```python
from build123d import *

# Parameters (mm, degrees)
BOX002_W          = 1
BOX002_H          = 6.4
BOX002_DEPTH      = 1.5
BOX006_W          = 10
BOX006_H          = 4.37
BOX006_DEPTH      = 12
BOX005_W          = 10
BOX005_H          = 4.37
BOX005_DEPTH      = 12
CYLINDER008_R     = 0.59
CYLINDER008_DEPTH = 50
CYLINDER009_R     = 0.59
CYLINDER009_DEPTH = 50
CYLINDER007_R     = 0.59
CYLINDER007_DEPTH = 50
BOX003_W          = 10
BOX003_H          = 4.37
BOX003_DEPTH      = 26
BOX004_W          = 10
BOX004_H          = 4.37
BOX004_DEPTH      = 26
BOX001_W          = 10
BOX001_H          = 5.5
BOX001_DEPTH      = 27
CYLINDER006_R     = 1.695
CYLINDER006_DEPTH = 20
CYLINDER003_R     = 1.1
CYLINDER003_DEPTH = 2
BOX_W             = 2
BOX_H             = 10
BOX_DEPTH         = 27.9
CYLINDER004_R     = 3
CYLINDER004_DEPTH = 27.4
CYLINDER005_R     = 1
CYLINDER005_DEPTH = 5.5
CYLINDER002_R     = 0.75
CYLINDER002_DEPTH = 6.2
CYLINDER001_R     = 2.5
CYLINDER001_DEPTH = 18
CYLINDER_R        = 2.2
CYLINDER_DEPTH    = 21.5


with BuildPart() as obj1:
    # Box002 → Box002 (new body)
    with BuildSketch(Plane(origin=(-0.5, -3.2, 21.5), x_dir=(1, 0, 0), z_dir=(0, 0, 1))):
        with Locations((0.5, 3.2)):
            Rectangle(BOX002_W, BOX002_H)
    extrude(amount=BOX002_DEPTH)


with BuildPart() as obj2:
    # Box006 → Box006 (new body)
    with BuildSketch(Plane(origin=(-10.25, -2.19, 36.77), x_dir=(1, 0, 0), z_dir=(0, 0, 1))):
        with Locations((5, 2.185)):
            Rectangle(BOX006_W, BOX006_H)
    extrude(amount=BOX006_DEPTH)


with BuildPart() as fusion004:
    # Box005 → Box005 (new body)
    with BuildSketch(Plane(origin=(0.25, -2.19, 36.77), x_dir=(1, 0, 0), z_dir=(0, 0, 1))):
        with Locations((5, 2.185)):
            Rectangle(BOX005_W, BOX005_H)
    extrude(amount=BOX005_DEPTH)

    # Fusion004: union obj2
    add(obj2.part)


with BuildPart() as fusion004_1:
    # Fusion004 placement: moved
    add(fusion004.part.moved(Location((0, 0, 1))))


with BuildPart() as m1_6_thread2:
    # Cylinder008 → Cylinder008 (new body)
    with BuildSketch(Plane(origin=(-4, 0, 29.41), x_dir=(0, 0, -1), z_dir=(1, 0, 0))):
        Circle(CYLINDER008_R)
    extrude(amount=CYLINDER008_DEPTH)


with BuildPart() as m1_6_thread3:
    # Cylinder009 → Cylinder009 (new body)
    with BuildSketch(Plane(origin=(-4, 0, 27.41), x_dir=(0, 0, -1), z_dir=(1, 0, 0))):
        Circle(CYLINDER009_R)
    extrude(amount=CYLINDER009_DEPTH)


with BuildPart() as mirrormountingholes:
    # Cylinder007 → Cylinder007 (new body)
    with BuildSketch(Plane(origin=(-4, 0, 31.405), x_dir=(0, 0, -1), z_dir=(1, 0, 0))):
        Circle(CYLINDER007_R)
    extrude(amount=CYLINDER007_DEPTH)

    # Fusion003: union M1_6__Thread2, M1_6__Thread3
    add(m1_6_thread2.part)
    add(m1_6_thread3.part)


with BuildPart() as obj3:
    # Box003 → Box003 (new body)
    with BuildSketch(Plane(origin=(0.5, -2.19, 23), x_dir=(1, 0, 0), z_dir=(0, 0, 1))):
        with Locations((5, 2.185)):
            Rectangle(BOX003_W, BOX003_H)
    extrude(amount=BOX003_DEPTH)


with BuildPart() as mirrorgrooves:
    # Box004 → Box004 (new body)
    with BuildSketch(Plane(origin=(-10.5, -2.19, 23), x_dir=(1, 0, 0), z_dir=(0, 0, 1))):
        with Locations((5, 2.185)):
            Rectangle(BOX004_W, BOX004_H)
    extrude(amount=BOX004_DEPTH)

    # Fusion002: union obj3
    add(obj3.part)


with BuildPart() as obj4:
    # Box001 → Box001 (new body)
    with BuildSketch(Plane(origin=(1, -2.57, 21), x_dir=(1, 0, 0), z_dir=(0, 0, 1))):
        with Locations((5, 2.75)):
            Rectangle(BOX001_W, BOX001_H)
    extrude(amount=BOX001_DEPTH)


with BuildPart() as probehole:
    # Cylinder006 → Cylinder006 (new body)
    with BuildSketch(Plane(origin=(-4, 0, 35.2), x_dir=(0, 0, -1), z_dir=(1, 0, 0))):
        Circle(CYLINDER006_R)
    extrude(amount=CYLINDER006_DEPTH)


with BuildPart() as beamhole:
    # Cylinder003 → Cylinder003 (new body)
    with BuildSketch(Plane(origin=(-1, 0, 35.2), x_dir=(0, 0, -1), z_dir=(1, 0, 0))):
        Circle(CYLINDER003_R)
    extrude(amount=CYLINDER003_DEPTH)


with BuildPart() as obj5:
    # Box → Box (new body)
    with BuildSketch(Plane(origin=(-1, -5, 21), x_dir=(1, 0, 0), z_dir=(0, 0, 1))):
        with Locations((1, 5)):
            Rectangle(BOX_W, BOX_H)
    extrude(amount=BOX_DEPTH)


with BuildPart() as cut004:
    # Cylinder004 → Cylinder004 (new body)
    with BuildSketch(Plane.XY.offset(21.5)):
        Circle(CYLINDER004_R)
    extrude(amount=CYLINDER004_DEPTH)

    # Common: intersect obj5
    add(obj5.part, mode=Mode.INTERSECT)

    # Cut001: cut BeamHole
    add(beamhole.part, mode=Mode.SUBTRACT)

    # Cut003: cut ProbeHole
    add(probehole.part, mode=Mode.SUBTRACT)

    # Cut004: cut obj4
    add(obj4.part, mode=Mode.SUBTRACT)


with BuildPart() as zylinder005:
    # Cylinder005 → Cylinder005 (new body)
    with BuildSketch(Plane.XY.offset(-0.5)):
        Circle(CYLINDER005_R)
    extrude(amount=CYLINDER005_DEPTH)


with BuildPart() as zylinder002:
    # Cylinder002 → Cylinder002 (new body)
    with BuildSketch(Plane(origin=(-3.25, 0, 2.95), x_dir=(0, 0, -1), z_dir=(1, 0, 0))):
        Circle(CYLINDER002_R)
    extrude(amount=CYLINDER002_DEPTH)


with BuildPart() as zylinder001:
    # Cylinder001 → Cylinder001 (new body)
    with BuildSketch(Plane.XY.offset(5)):
        Circle(CYLINDER001_R)
    extrude(amount=CYLINDER001_DEPTH)


with BuildPart() as fusion005:
    # Cylinder → Cylinder (new body)
    with BuildSketch(Plane.XY.offset(-0.5)):
        Circle(CYLINDER_R)
    extrude(amount=CYLINDER_DEPTH)

    # Fusion: union Zylinder001
    add(zylinder001.part)

    # Cut: cut Zylinder002
    add(zylinder002.part, mode=Mode.SUBTRACT)

    # Cut002: cut Zylinder005
    add(zylinder005.part, mode=Mode.SUBTRACT)

    # Fusion001: union Cut004
    add(cut004.part)

    # Cut005: cut MirrorGrooves
    add(mirrorgrooves.part, mode=Mode.SUBTRACT)

    # Cut006: cut MirrorMountingHoles
    add(mirrormountingholes.part, mode=Mode.SUBTRACT)

    # Cut007: cut Fusion004
    add(fusion004_1.part, mode=Mode.SUBTRACT)

    # Fusion005: union obj1
    add(obj1.part)


solid = fusion005.part
```
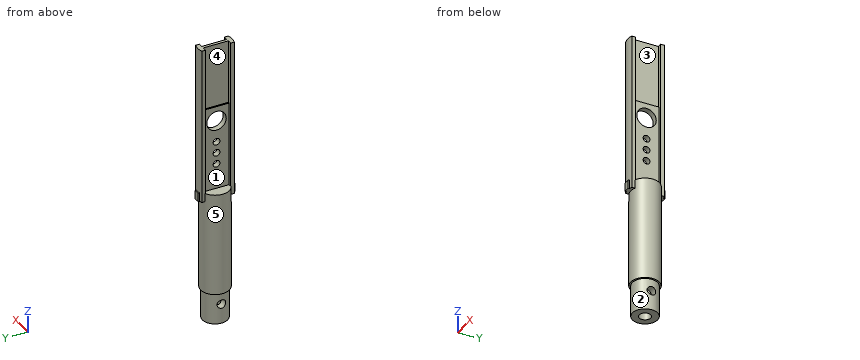
Verification items for the finished model (mm, model axes). Face numbers are marked on the shaded views. A direction names the side the tool comes from. Give positions to 0.01 mm unless a question says otherwise; leave off trailing zeros. Loops run counter-clockwise (first coordinate to the right, second up) from the corner with the lowest first, then second, coordinate; pieces in that order, holes last.
1. Section check C-C, the plane y = 0. Count the separate pieces of the cut face and the enclosed holes in it, then the cut area to 3 significant figures.
2. Section check A-A, the plane z = 29.41. Enter the section's corners in (x, y).
3. Section check D-D, the plane x = 1.55. Enter the section's corners in (y, z), then the cut area to 3 significant figures.
4. Go/stop test with flat-tipped pins: pin 1 Ø2 at (y, z) = (-1, 32.5) entering from +X; pin 2 Ø0.6 at (x, z) = (0.5, 32) entering from +Y; pin 3 Ø1.5 at (x, z) = (0, 15.5) entering from -Y. Record where each tip stops, or that it passes through.
5. Set-up check for the marked faces 3, 4 and 5: record each of +Z, -Z, +X, -X, +Y, -Y from which the full face is reachable in a straight line by a thin tool's end or side.
6. Mould release check, pull along Y, two halves, no side actions. Record for the marked faces 1 and 2: released by +Y, released by -Y, zero draft, split by the parting line, or undercut.
7. Thickness scan on line 1 (Z direction, x = 0.35, y = 0) (3 decimals); line 2 (Y direction, x = 0, z = 3.2); line 3 (Y direction, x = -0.2, z = 35.2) (3 decimals). Record the ranges inside material, lowest first.
8. Section check B-B, the plane z = 44. Enter the section's corners in (x, y).
Geometry says:
1. separate pieces: 7
1. enclosed holes: 0
1. area: 113 mm2
2. outline: (-1, -2.83) arc R3 ccw to (1, -2.83) - (1, -2.19) - (0.5, -2.19) - (0.5, -0.59) - (-0.5, -0.59) - (-0.5, -2.19) - (-1, -2.19) - close; (-1, 2.18) - (-0.5, 2.18) - (-0.5, 0.59) - (0.5, 0.59) - (0.5, 2.18) - (1, 2.18) - (1, 2.83) arc R3 ccw to (-1, 2.83) - close
3. outline: (-1.96, 5) - (-1.56, 5) - (-1.56, -0.5) - (1.56, -0.5) - (1.56, 5) - (1.96, 5) - (1.96, 23) - (-1.96, 23) - close; hole circle Ø1.5 at (0, 2.95)
3. area: 86.0 mm2
4. pin 1: stops at x = 0.5
4. pin 2: stops at y = 2.99
4. pin 3: stops at y = -2.5
5. face 3: +Z, +X
5. face 4: +Z, -X
5. face 5: -Z
6. face 1: undercut
6. face 2: split by the parting line
7. line 1: z = 5 to 26.82, 28 to 28.82, 30 to 30.815, 31.995 to 33.505, 36.895 to 37.77
7. line 2: y = -2.2 to -1, 1 to 2.2
7. line 3: y = -2.993 to -1.695, 1.695 to 2.993
8. outline: (-1, -2.83) arc R3 ccw to (1, -2.83) - (1, -2.19) - (0.25, -2.19) - (0.25, 2.18) - (1, 2.18) - (1, 2.83) arc R3 ccw to (-1, 2.83) - (-1, 2.18) - (-0.25, 2.18) - (-0.25, -2.19) - (-1, -2.19) - close
